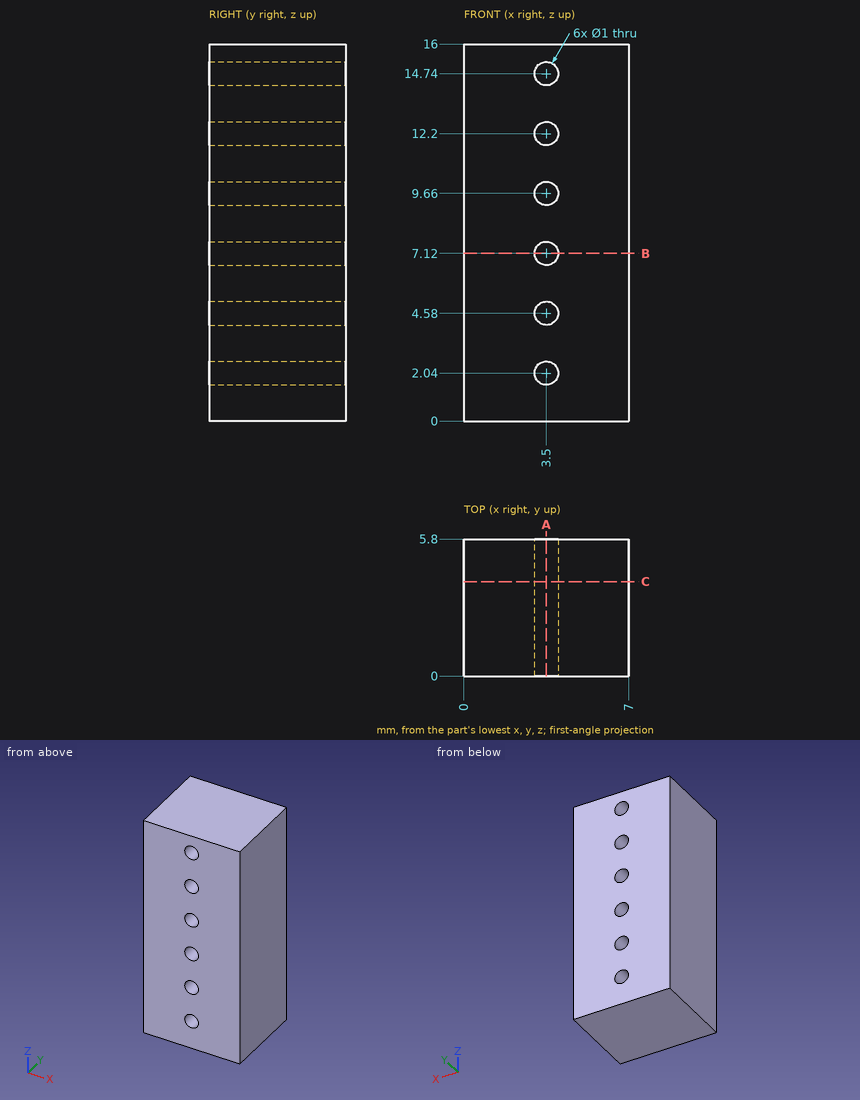
Here's the drawing with two shaded views (mm, measured from the low corner). I have some questions. Round coordinates to 2 decimals unless told otherwise and drop trailing zeros. Write each loop counter-clockwise with the first axis right and the second up, starting at its lowest first coordinate (ties: lowest second). Pieces come first, ordered by that corner, then holes. Notation, with made-up numbers: M 9,49.25 L 58,49.25 A15 cw 58,76.25 Z; hole C 46.5,-15.75 d11. An arc over 180 degrees is marked long. Answer in a Markdown table with one row per item. Add a question column.
Q1. Imagine slicing it at B-B (z = 7.12). Please give me the cut outline in (x, y), then the cut area to 3 significant figures.
Q2. Imagine slicing it at A-A (x = 3.5). Please give me the cut outline in (y, z), then the cut area to 3 significant figures.
Q3. If I drill on line 1 (X direction, y = 2, z = 7.12), over which ranges is the centre line in solid material (lowest first)? Write a range as from..to.
Q4. Imagine slicing it at C-C (y = 4). Please give me the cut outline in (x, z), then the cut area to 3 significant figures.
Values:
| question | item | result |
|---|---|---|
| 1 | outline | M 0,0 L 3,0 L 3,5.8 L 0,5.8 Z; M 4,0 L 7,0 L 7,5.8 L 4,5.8 Z |
| 1 | area | 34.8 mm^2 |
| 2 | outline | M 0,0 L 5.8,0 L 5.8,1.54 L 0,1.54 Z; M 0,2.54 L 5.8,2.54 L 5.8,4.08 L 0,4.08 Z; M 0,5.08 L 5.8,5.08 L 5.8,6.62 L 0,6.62 Z; M 0,7.62 L 5.8,7.62 L 5.8,9.16 L 0,9.16 Z; M 0,10.16 L 5.8,10.16 L 5.8,11.7 L 0,11.7 Z; M 0,12.7 L 5.8,12.7 L 5.8,14.24 L 0,14.24 Z; M 0,15.24 L 5.8,15.24 L 5.8,16 L 0,16 Z |
| 2 | area | 58.0 mm^2 |
| 3 | line 1 | 0..3, 4..7 |
| 4 | outline | M 0,0 L 7,0 L 7,16 L 0,16 Z; hole C 3.5,2.04 d1; hole C 3.5,4.58 d1; hole C 3.5,7.12 d1; hole C 3.5,9.66 d1; hole C 3.5,12.2 d1; hole C 3.5,14.74 d1 |
| 4 | area | 107 mm^2 |
